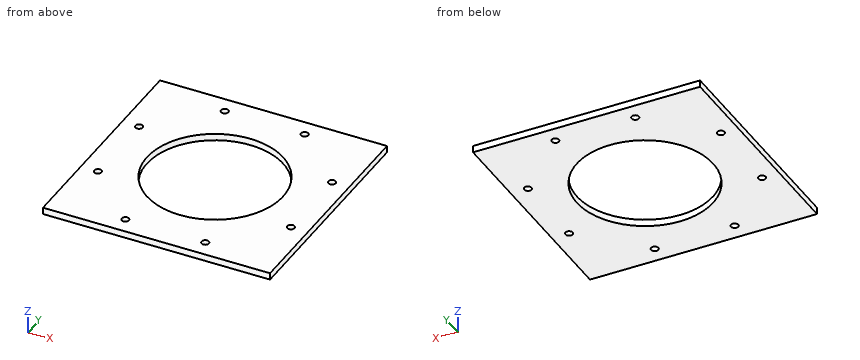
Autodesk Inventor part; units mm, degrees
ref_plane "YZ Plane" through (0, 0, 0) normal (1, 0, 0) x (0, 1, 0)
ref_plane "XZ Plane" through (0, 0, 0) normal (0, 1, 0) x (-1, 0, 0)
ref_plane "XY Plane" through (0, 0, 0) normal (0, 0, 1) x (1, 0, 0)
sketch "スケッチ1" plane through (0, 0, 0) normal (0, 0, 1) x (1, 0, 0)
  line L0 (-50, 50) -> (50, 50)
  line L1 (50, 50) -> (50, -50)
  line L2 (50, -50) -> (-50, -50)
  line L3 (-50, -50) -> (-50, 50)
  line L4 (0, 0) -> (0, 50) construction
  line L5 (0, 0) -> (50, 0) construction
  dimension "d0" = 100
  dimension "d1" = 100
extrude "押し出し1" add sketch "スケッチ1" along normal blind 3
sketch "スケッチ2" plane through (0, 0, 3) normal (0, 0, 1) x (1, 0, 0)
  point P0 (0, 0)
  point P1 (0, 0)
hole "穴1" at (0, 0, 3) direction (0, 0, -1) diameter 60 end through all
sketch "スケッチ3" plane through (0, 0, 3) normal (0, 0, 1) x (1, 0, 0)
  line L0 (0, 0) -> (0, 50) construction
  line L1 (50, 50) -> (-50, 50)
  line L2 (0, 0) -> (19.8012, 47.8043) construction
  point P0 (17.6034, 42.4985)
  point P1 (-17.6034, 42.4985)
  point P2 (-42.4985, 17.6034)
  point P3 (-42.4985, -17.6034)
  point P4 (-17.6034, -42.4985)
  point P5 (17.6034, -42.4985)
  point P6 (42.4985, -17.6034)
  point P7 (42.4985, 17.6034)
  dimension "d11" = 22.5
  dimension "d12" = 46
  dimension "d15" = 360
hole "穴2" at (17.6034, 42.4985, 3) at (-17.6034, 42.4985, 3) at (-42.4985, 17.6034, 3) at (-42.4985, -17.6034, 3) at (-17.6034, -42.4985, 3) at (17.6034, -42.4985, 3) at (42.4985, -17.6034, 3) at (42.4985, 17.6034, 3) direction (0, 0, -1) diameter 3.2 end through all
properties part number "base_plate" material "アルミニウム 6061"
The listing builds one solid part. Answer for the finished solid, in the listing's coordinates (mm). Coordinates: 2 decimals unless noted, no trailing zeros. Order: outer loops, then holes, each group sorted by start corner. A loop starts at its lowest first (then second) coordinate and runs counter-clockwise, first axis right, second up. Notation, with made-up numbers: (51.5, 51.5) -> (89.5, 51.5) arc R32 cw to (89.5, 87.5) -> close; hole circle Ø9 at (-17.75, 25). An arc over 180 degrees is marked (long way). Answer in a Markdown table with one row per item. Add a question column.
Item 1: Find the intervals of material crossed by L1, parallel to X at y = 41.5, z = 1.55; L2, parallel to X at y = 43, z = 0.4; L3, parallel to Y at x = 17, z = 2.5, in increasing order. Write a range as from..to.
Item 2: Find section A-A (y = 0). Write down the section's boundary in (x, z), then the cut area to 3 significant figures.
Item 3: Find section C-C (z = 0.45). State how many separate pieces and enclosed holes the cut face has, then the cut area to 3 significant figures.
Result set:
| question | item | result |
|---|---|---|
| 1 | L1 | x = -50..-18.85, -16.35..16.35, 18.85..50 |
| 1 | L2 | x = -50..-19.12, -16.08..16.08, 19.12..50 |
| 1 | L3 | y = -50..-43.98, -41.02..-24.72, 24.72..41.02, 43.98..50 |
| 2 | outline | (-50, 0) -> (-30, 0) -> (-30, 3) -> (-50, 3) -> close; (30, 0) -> (50, 0) -> (50, 3) -> (30, 3) -> close |
| 2 | area | 120 mm² |
| 3 | separate pieces | 1 |
| 3 | enclosed holes | 9 |
| 3 | area | 7,110 mm² |
